from build123d import *

# Parameters (mm, degrees)
F0_R     = 114.3
F0_R_2   = 3.175
F1_DEPTH = 12.7
F2_R     = 9.525
F2_R_2   = 3.175
F3_DEPTH = 39.878
F4_SIZE  = 2.38125
F5_SIZE  = 1.5875
F6_SIZE  = 1.5875


with BuildPart() as f1:
    # F0 (on Top) → F1 (new body)
    with BuildSketch(Plane.XY):
        Circle(F0_R)
        with Locations((-69.85, 0)):
            Circle(F0_R_2, mode=Mode.SUBTRACT)
    extrude(amount=F1_DEPTH)

    # F2 (on face) → F3 (join)
    with BuildSketch(Plane.XY.offset(12.7)):
        with BuildLine():
            ThreePointArc((76.2, 0), (69.85, 6.35), (63.5, 0))
            ThreePointArc((63.5, 0), (69.85, -6.35), (76.2, 0))
        make_face()
        with Locations((-69.85, 0)):
            Circle(F2_R)
        with Locations((-69.85, 0)):
            Circle(F2_R_2, mode=Mode.SUBTRACT)
    extrude(amount=F3_DEPTH)

    # F4
    f4_edges = [f1.edges().sort_by_distance(p)[0] for p in [
        (-73.025, 0, 52.578),
    ]]
    chamfer(f4_edges, length=F4_SIZE)

    # F5
    f5_edges = [f1.edges().sort_by_distance(p)[0] for p in [
        (76.2, 0, 52.578),
    ]]
    chamfer(f5_edges, length=F5_SIZE)

    # F6
    f6_edges = [f1.edges().sort_by_distance(p)[0] for p in [
        (-79.375, 0, 52.578),
    ]]
    chamfer(f6_edges, length=F6_SIZE)


solid = f1.part
The model under review builds one solid part; all positions refer to its coordinate system, in mm. A direction names the side the tool comes from. Give positions to 0.01 mm unless a question says otherwise; leave off trailing zeros. Loops run counter-clockwise (first coordinate to the right, second up) from the corner with the lowest first, then second, coordinate; pieces in that order, holes last. Notation, with made-up numbers: (68, 78.25) -> (82, 78.25) arc R10 cw to (82, 95.25) -> close; hole circle Ø8 at (6.25, 79). An arc over 180 degrees is marked (long way). Put each result on its own line as item: value. Start each with the question number.
1. We need section C-C on z = 32.5. State the section outline as (x, y) points (3 decimals).
2. For faces 1 (the face through (-79.366, 0.419, 31.577)), 2 (the face through (70, 0, 52.578)), list the 3-axis set-ups (+Z, -Z, +X, -X, +Y, -Y) from which the entire face can be reached by the end or side of a thin tool; tool diameter is ignored.
3. We need section A-A on y = 0. State the section outline as (x, z) points (1 decimal).
4. Wall thickness on probe 1 along Y at (x, z) = (-69.85, 17.5) (3 decimals); probe 2 along Z at (x, y) = (-15.5, 89); probe 3 along Y at (x, z) = (-69, 19): over which ranges is each line inside the solid? List them lowest first.
5. Clearance check with flat-ended pins moving along their axes: P1, Ø5, axis at x = 21, y = -10.5, coming from the -Z side; P2, Ø3, axis at x = 31.5, y = 61.5, coming from the +Z side; P3, Ø5, axis at x = -69.85, y = 0, coming from the +Z side; P4, Ø3, axis at x = 67.5, z = 39, coming from the +Y side. State where each tip first meets the part, or that it passes through.
6. We need section D-D on x = 0. State the section outline as (y, z) points, then the cut area to 3 significant figures.
7. We need section B-B on x = -69.85. State the section outline as (y, z) points (1 decimal), then the cut area to 3 significant figures.
Determined:
1. outline: circle Ø19.05 at (-69.85, 0); circle Ø12.7 at (69.85, 0); hole circle Ø6.35 at (-69.85, 0)
2. face 1: +Z
2. face 2: +Z, +X, -X, +Y, -Y
3. outline: (-114.3, 0) -> (-73, 0) -> (-73, 50.2) -> (-75.4, 52.6) -> (-77.8, 52.6) -> (-79.4, 51) -> (-79.4, 12.7) -> (-114.3, 12.7) -> close; (-66.7, 0) -> (114.3, 0) -> (114.3, 12.7) -> (76.2, 12.7) -> (76.2, 51) -> (74.6, 52.6) -> (65.1, 52.6) -> (63.5, 51) -> (63.5, 12.7) -> (-60.3, 12.7) -> (-60.3, 51) -> (-61.9, 52.6) -> (-64.3, 52.6) -> (-66.7, 50.2) -> close
4. probe 1: -9.525 to -3.175, 3.175 to 9.525
4. probe 2: 0 to 12.7
4. probe 3: -9.49 to -3.06, 3.06 to 9.49
5. P1: z = 0
5. P2: z = 12.7
5. P3: through
5. P4: y = 6.29
6. outline: (-114.3, 0) -> (114.3, 0) -> (114.3, 12.7) -> (-114.3, 12.7) -> close
6. area: 2,900 mm^2
7. outline: (-90.5, 0) -> (-3.2, 0) -> (-3.2, 50.2) -> (-5.6, 52.6) -> (-7.9, 52.6) -> (-9.5, 51) -> (-9.5, 12.7) -> (-90.5, 12.7) -> close; (3.2, 0) -> (90.5, 0) -> (90.5, 12.7) -> (9.5, 12.7) -> (9.5, 51) -> (7.9, 52.6) -> (5.6, 52.6) -> (3.2, 50.2) -> close
7. area: 2,720 mm^2
